from build123d import *

# Parameters (mm, degrees)
F1_DEPTH = 3
F2_R     = 2
F3_DEPTH = 25
F4_R     = 1.5
F5_DEPTH = 25


with BuildPart() as f1:
    # F0 (on Top) → F1 (new body)
    with BuildSketch(Plane.XY):
        with BuildLine():
            Line((80.619057, -25.905496), (-116.380943, -25.905496))
            ThreePointArc((-116.380943, -25.905496), (-118.502264, -26.784176), (-119.380943, -28.905496))
            Line((-119.380943, -28.905496), (-119.380943, -275.905496))
            ThreePointArc((-119.380943, -275.905496), (-118.502264, -278.026816), (-116.380943, -278.905496))
            Line((-116.380943, -278.905496), (80.619057, -278.905496))
            ThreePointArc((80.619057, -278.905496), (82.740377, -278.026816), (83.619057, -275.905496))
            Line((83.619057, -275.905496), (83.619057, -28.905496))
            ThreePointArc((83.619057, -28.905496), (82.740377, -26.784176), (80.619057, -25.905496))
        make_face()
        with BuildLine():
            ThreePointArc((-89.380943, -56.905496), (-88.502264, -54.784176), (-86.380943, -53.905496))
            Line((-86.380943, -53.905496), (50.619057, -53.905496))
            ThreePointArc((50.619057, -53.905496), (52.740377, -54.784176), (53.619057, -56.905496))
            Line((53.619057, -56.905496), (53.619057, -247.905496))
            ThreePointArc((53.619057, -247.905496), (52.740377, -250.026816), (50.619057, -250.905496))
            Line((50.619057, -250.905496), (-86.380943, -250.905496))
            ThreePointArc((-86.380943, -250.905496), (-88.502264, -250.026816), (-89.380943, -247.905496))
            Line((-89.380943, -247.905496), (-89.380943, -56.905496))
        make_face(mode=Mode.SUBTRACT)
    extrude(amount=F1_DEPTH)

    # F2 (on face) → F3 (cut)
    with BuildSketch(Plane.XY.offset(3)):
        with Locations((-109.880943, -63.905496)):
            Circle(F2_R)
        with Locations((74.119057, -63.905496)):
            Circle(F2_R)
        with Locations((74.119057, -152.405496)):
            Circle(F2_R)
        with Locations((74.119057, -240.905496)):
            Circle(F2_R)
        with Locations((-109.880943, -240.905496)):
            Circle(F2_R)
        with Locations((-109.880943, -152.405496)):
            Circle(F2_R)
    extrude(amount=-F3_DEPTH, mode=Mode.SUBTRACT)

    # F4 (on face) → F5 (cut)
    with BuildSketch(Plane.XY.offset(3)):
        with Locations((-92.880943, -52.405496)):
            Circle(F4_R)
        with BuildLine():
            ThreePointArc((-17.880943, -50.405496), (-16.820283, -49.966156), (-16.380943, -48.905496))
            ThreePointArc((-16.380943, -48.905496), (-18.941603, -47.844836), (-17.880943, -50.405496))
        make_face()
        with Locations((57.119057, -52.405496)):
            Circle(F4_R)
        with Locations((57.119057, -102.405496)):
            Circle(F4_R)
        with Locations((-92.880943, -102.405496)):
            Circle(F4_R)
        with Locations((57.119057, -152.405496)):
            Circle(F4_R)
        with Locations((-92.880943, -152.405496)):
            Circle(F4_R)
        with Locations((-92.880943, -202.405496)):
            Circle(F4_R)
        with Locations((57.119057, -202.405496)):
            Circle(F4_R)
        with Locations((-92.880943, -252.405496)):
            Circle(F4_R)
        with BuildLine():
            ThreePointArc((-17.880943, -254.405496), (-18.941603, -256.966156), (-16.380943, -255.905496))
            ThreePointArc((-16.380943, -255.905496), (-16.820283, -254.844836), (-17.880943, -254.405496))
        make_face()
        with Locations((57.119057, -252.405496)):
            Circle(F4_R)
    extrude(amount=-F5_DEPTH, mode=Mode.SUBTRACT)


solid = f1.part
Read the model definition and answer for the solid it produces. Units are mm, in the model's axes. Give positions to 0.01 mm unless a question says otherwise; leave off trailing zeros. Write each loop counter-clockwise with the first axis right and the second up, starting at its lowest first coordinate (ties: lowest second). Pieces come first, ordered by that corner, then holes. Notation, with made-up numbers: (2, -31.5) - (52, -31.5) arc R35 cw to (52, 4.5) - close; hole circle Ø2 at (-33, 68). An arc over 180 degrees is marked (long way). Return JSON: item names as keys, results as strings.
Q1. A cutting plane is placed at C-C, the plane z = 2.25. Count the separate pieces of the cut face and the enclosed holes in it, and give its area (3 significant figures).
Reply:
{"separate pieces": "1", "enclosed holes": "19", "area": "23,000 mm²"}
Q2. A cutting plane is placed at A-A, the plane x = 45.5. Determine the outline of the cut face in (y, z), and give its area (3 significant figures).
Reply:
{"outline": "(-278.91, 0) - (-250.91, 0) - (-250.91, 3) - (-278.91, 3) - close; (-53.91, 0) - (-25.91, 0) - (-25.91, 3) - (-53.91, 3) - close", "area": "168 mm²"}
Q3. A cutting plane is placed at B-B, the plane y = -228.5. Determine the outline of the cut face in (x, z).
Reply:
{"outline": "(-119.38, 0) - (-89.38, 0) - (-89.38, 3) - (-119.38, 3) - close; (53.62, 0) - (83.62, 0) - (83.62, 3) - (53.62, 3) - close"}
Q4. Consider line 1 along Y through (x, z) = (11.5, 2.2); line 2 along X through (y, z) = (-68.5, 2.1); line 3 along Y through (x, z) = (-109, 1.9). Determine where each line is inside the solid, lowest interval first. Write a range as [from, to].
Reply:
{"line 1": "[-278.91, -250.91], [-53.91, -25.91]", "line 2": "[-119.38, -89.38], [53.62, 83.62]", "line 3": "[-278.91, -242.7], [-239.11, -154.2], [-150.61, -65.7], [-62.11, -25.91]"}
Q5. Given P1, Ø1.8, axis at x = 57.12, y = -52.41, coming from the +Z side, flat-ended and moving along its own axis, determine where the tip first touches the part or whether it passes through.
Reply:
{"P1": "through"}
